from build123d import *

# Parameters (mm, degrees)
SKETCH_W        = 56
SKETCH_H        = 25
PAD_DEPTH       = 2
SKETCH001_W     = 2
SKETCH001_H     = 25
PAD001_DEPTH    = 62
SKETCH002_R     = 4
SKETCH002_R_2   = 1.5
POCKET_DEPTH    = 56.001
FILLET_R        = 12.499
FILLET001_R     = 1.99
SKETCH003_R     = 4
SKETCH003_R_2   = 1.5
POCKET001_DEPTH = 5


with BuildPart() as part:
    # Sketch → Pad (new body)
    with BuildSketch(Plane.XY):
        Rectangle(SKETCH_W, SKETCH_H)
    extrude(amount=PAD_DEPTH)

    # Sketch001 (on Face6 of Pad) → Pad001 (join)
    with BuildSketch(Plane.XY.offset(2)):
        with Locations((27, 0)):
            Rectangle(SKETCH001_W, SKETCH001_H)
        with Locations((-27, 0)):
            Rectangle(SKETCH001_W, SKETCH001_H)
    extrude(amount=PAD001_DEPTH)

    # Sketch002 (on Face10 of Pad001) → Pocket (cut, through all)
    with BuildSketch(Plane.YZ.offset(28)):
        with Locations((0, 53.5)):
            Circle(SKETCH002_R)
        with Locations((0, 47)):
            Circle(SKETCH002_R_2)
        with Locations((6.5, 53.5)):
            Circle(SKETCH002_R_2)
        with Locations((-6.5, 53.5)):
            Circle(SKETCH002_R_2)
        with Locations((0, 60)):
            Circle(SKETCH002_R_2)
    extrude(amount=-POCKET_DEPTH, mode=Mode.SUBTRACT)

    # Fillet
    fillet_edges = [part.edges().sort_by_distance(p)[0] for p in [
        (-27, -12.5, 64),
        (-27, 12.5, 64),
        (27, -12.5, 64),
        (27, 12.5, 64),
    ]]
    fillet(fillet_edges, radius=FILLET_R)

    # Fillet001
    fillet001_edges = [part.edges().sort_by_distance(p)[0] for p in [
        (28, 0, 0),
        (-28, 0, 0),
    ]]
    fillet(fillet001_edges, radius=FILLET001_R)

    # Sketch003 (on Face6 of Fillet001) → Pocket001 (cut)
    with BuildSketch(Plane.XY.offset(2)):
        Circle(SKETCH003_R)
        with Locations((6.5, 0)):
            Circle(SKETCH003_R_2)
        with Locations((-6.5, 0)):
            Circle(SKETCH003_R_2)
        with Locations((0, -6.5)):
            Circle(SKETCH003_R_2)
        with Locations((0, 6.5)):
            Circle(SKETCH003_R_2)
    extrude(amount=-POCKET001_DEPTH, mode=Mode.SUBTRACT)


solid = part.part
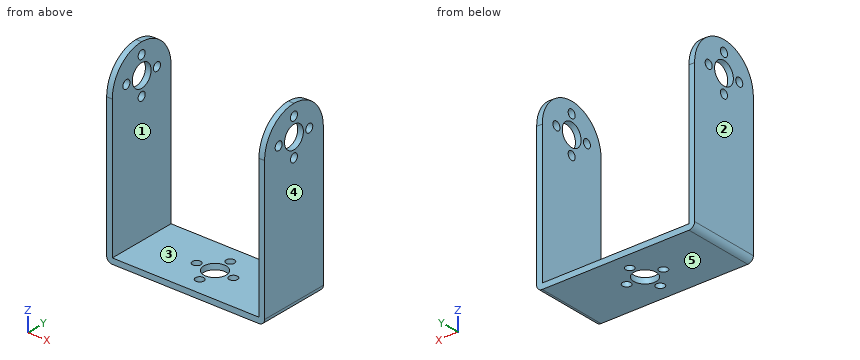
The model under review builds one solid part; all positions refer to its coordinate system, in mm. Face numbers are marked on the shaded views. A direction names the side the tool comes from. Round coordinates to 2 decimals unless told otherwise and drop trailing zeros. Loops run counter-clockwise (first coordinate to the right, second up) from the corner with the lowest first, then second, coordinate; pieces in that order, holes last. Notation, with made-up numbers: (40.5, 76) -> (49.5, 76) arc R21 cw to (49.5, 88) -> close; hole circle Ø11 at (-15.75, 89). An arc over 180 degrees is marked (long way). Write item = value, one per line. Start each with the question number.
Item 1: Take a section at B-B on z = 33.5. Give the boundary of the cut face in (x, y), plus the area to 3 significant figures.
Item 2: To check wall thickness, follow L1, parallel to X at y = 0.75, z = 22.5; L2, parallel to Y at x = 0, z = 1.1; L3, parallel to Z at x = -27.45, y = 0. State the ranges of each line that lie inside material, in increasing order.
Item 3: For the marked faces 1 and 2, list the 3-axis set-ups (+Z, -Z, +X, -X, +Y, -Y) from which the entire face can be reached by the end or side of a thin tool; tool diameter is ignored.
Item 4: Insertion check: pin 1 (2.5 mm diameter, centred on y = 0, z = 47, fed in from -X); pin 2 (5 mm diameter, centred on x = 0, y = 6.5, fed in from +Z). Each pin has a flat end and moves straight along its axis. Give the tip position at first contact, or say it passes through.
Item 5: Mouldability with a two-part tool opening along X and no side actions: class the marked faces 3, 4 and 5 as released by +X, released by -X, zero draft, split by the parting line, or undercut.
Item 6: Take a section at D-D on x = 0. Give the boundary of the cut face in (y, z), plus the area to 3 significant figures.
Item 7: Take a section at A-A on x = 6.5. Give the boundary of the cut face in (y, z), plus the area to 3 significant figures.
Item 8: Take a section at C-C on y = 6.5. Give the boundary of the cut face in (x, z), plus the area to 3 significant figures.
Result:
q1.outline = (-28, -12.5) -> (-26, -12.5) -> (-26, 12.5) -> (-28, 12.5) -> close; (26, -12.5) -> (28, -12.5) -> (28, 12.5) -> (26, 12.5) -> close
q1.area = 100 mm²
q2.L1 = -28 to -26, 26 to 28
q2.L2 = -12.5 to -8, -5 to -4, 4 to 5, 8 to 12.5
q2.L3 = 0.62 to 45.5, 48.5 to 49.5, 57.5 to 58.5, 61.5 to 64
q3.face_1 = +Z, +Y, -Y
q3.face_2 = +Z, -Z, -X, +Y, -Y
q4.pin_1 = through
q4.pin_2 = 2
q5.face_3 = undercut
q5.face_4 = released by +X
q5.face_5 = zero draft
q6.outline = (-12.5, 0) -> (-8, 0) -> (-8, 2) -> (-12.5, 2) -> close; (-5, 0) -> (-4, 0) -> (-4, 2) -> (-5, 2) -> close; (4, 0) -> (5, 0) -> (5, 2) -> (4, 2) -> close; (8, 0) -> (12.5, 0) -> (12.5, 2) -> (8, 2) -> close
q6.area = 22.0 mm²
q7.outline = (-12.5, 0) -> (-1.5, 0) -> (-1.5, 2) -> (-12.5, 2) -> close; (1.5, 0) -> (12.5, 0) -> (12.5, 2) -> (1.5, 2) -> close
q7.area = 44.0 mm²
q8.outline = (-28, 1.99) arc R1.99 ccw to (-26.01, 0) -> (-1.5, 0) -> (-1.5, 2) -> (-26, 2) -> (-26, 52) -> (-28, 52) -> close; (-28, 55) -> (-26, 55) -> (-26, 62.18) -> (-28, 62.18) -> close; (1.5, 0) -> (26.01, 0) arc R1.99 ccw to (28, 1.99) -> (28, 52) -> (26, 52) -> (26, 2) -> (1.5, 2) -> close; (26, 55) -> (28, 55) -> (28, 62.18) -> (26, 62.18) -> close
q8.area = 333 mm²
